Read the model definition and answer for the solid it produces. Units are mm, in the model's axes. A direction names the side the tool comes from. Coordinates: 2 decimals unless noted, no trailing zeros. Loops run counter-clockwise (first coordinate to the right, second up) from the corner with the lowest first, then second, coordinate; pieces in that order, holes last.
from build123d import *

# Parameters (mm, degrees)
SKETCH8_W           = 26
SKETCH8_H           = 10
BOSS_EXTRUDE5_DEPTH = 190
SKETCH9_R           = 6.25
BOSS_EXTRUDE7_DEPTH = 28
SKETCH13_R          = 5
CUT_EXTRUDE3_DEPTH  = 28
SKETCH14_R          = 1.5
CUT_EXTRUDE4_DEPTH  = 28


with BuildPart() as part:
    # Sketch8 → Boss-Extrude5 (new body)
    with BuildSketch(Plane(origin=(0, 0, 0), x_dir=(1, 0, 0), z_dir=(0, 1, 0))):
        Rectangle(SKETCH8_W, SKETCH8_H)
    extrude(amount=BOSS_EXTRUDE5_DEPTH)

    # Sketch9 → Boss-Extrude7 (add)
    with BuildSketch(Plane(origin=(13, 0, 0), x_dir=(0, 0, -1), z_dir=(1, 0, 0))):
        with Locations((-0.118358798, -3.586767795)):
            Circle(SKETCH9_R)
    extrude(amount=-BOSS_EXTRUDE7_DEPTH)

    # Sketch13 → Cut-Extrude3 (cut)
    with BuildSketch(Plane(origin=(13, 0, 0), x_dir=(0, 0, -1), z_dir=(1, 0, 0))):
        with Locations((-0.118358798, -3.586767795)):
            Circle(SKETCH13_R)
    extrude(amount=-CUT_EXTRUDE3_DEPTH, mode=Mode.SUBTRACT)

    # Sketch14 → Cut-Extrude4 (cut)
    with BuildSketch(Plane(origin=(13, 0, 0), x_dir=(0, 0, -1), z_dir=(1, 0, 0))):
        with Locations((-0.059179399, 90.081616102)):
            Circle(SKETCH14_R)
    extrude(amount=-CUT_EXTRUDE4_DEPTH, mode=Mode.SUBTRACT)


solid = part.part
Q1. A cutting plane is placed at B-B (x = -4.25). Give the vertices of the cut face in (y, z).
Findings below:
outline: (0, -5) - (190, -5) - (190, 5) - (0.32, 5) arc R6.25 ccw (long way) to start; hole circle Ø10 at (-3.59, 0.12); hole circle Ø3 at (90.08, 0.06)
Q2. Straight lines are drawn through the part: probe 1 along Y at (x, z) = (-8.25, -1); probe 2 along Y at (x, z) = (9.75, 0.5); probe 3 along Z at (x, y) = (11.5, 2.5). For each, find the intervals that lie inside material, in ascending order.
Findings below:
probe 1: y = -9.74 to -8.46, 1.29 to 89.02, 91.14 to 190
probe 2: y = -9.83 to -8.57, 1.4 to 88.65, 91.52 to 190
probe 3: z = -5 to 5
Q3. Flat-ended cylindrical pins translate along their axes: pin 1 Ø2 at (x, y) = (6, 112) entering from +Z; pin 2 Ø13 at (x, y) = (-4, 82) entering from -Z; pin 3 Ø5 at (y, z) = (90.08, 0.06) entering from -X. Find the tip coordinate at first contact, or state that the pin passes through.
Findings below:
pin 1: stops at z = 5
pin 2: stops at z = -5
pin 3: stops at x = -13
Q4. A cutting plane is placed at A-A (y = 34). Give the vertices of the cut face in (x, z), then the cut area to 3 significant figures.
Findings below:
outline: (-13, -5) - (13, -5) - (13, 5) - (-13, 5) - close
area: 260 mm2
Q5. Determine the mould class of faces 3 (the face through (0, 190, 0)), 4 (the face through (-0.8, -2.08, -4.65)), 5 (the face through (0, 94, -5)) for opening direction Y: +Y half, -Y half, draft (parallel to the pull), parting line (faces both ways), or undercut.
Findings below:
face 3: +Y half
face 4: undercut
face 5: draft
Q6. Which of the six approach directions +Z, -Z, +X, -X, +Y, -Y give full straight-line access (tool end or side, diameter ignored) to faces 1 (the face through (0, 94, 5)), 2 (the face through (-15, 1, 3))?
Findings below:
face 1: +Z, +X, -X, +Y
face 2: +Z, -Z, -X, +Y, -Y
